```python
from build123d import *

# Parameters (mm, degrees)
SKETCH022_R        = 30
PAD_DEPTH          = 17
SKETCH023_R        = 0.7
POCKET_DEPTH       = 15.9
SKETCH024_R        = 0.55
POCKET001_DEPTH    = 13
SKETCH025_R        = 0.5
POCKET002_DEPTH    = 2
SKETCH026_W        = 5.1
SKETCH026_H        = 3.1
POCKET003_DEPTH    = 10
POLARPATTERN_COUNT = 3
SKETCH032_R        = 4
PAD002_DEPTH       = 7.5
SKETCH033_R        = 2.25
POCKET008_DEPTH    = 6
CHAMFER_SIZE       = 0.6
CHAMFER001_SIZE    = 0.8
SKETCH038_R        = 4.25
POCKET011_DEPTH    = 0.4
POCKET013_DEPTH    = 14
SKETCH046_W        = 4
SKETCH046_H        = 3
PAD010_DEPTH       = 14.5
CHAMFER006_SIZE    = 0.5
FILLET001_R        = 2


with BuildPart() as part:
    # Sketch022 (on DatumPlane) → Pad (new body)
    with BuildSketch(Plane(origin=(0, 0, -14.6), x_dir=(1, 0, 0), z_dir=(0, 0, -1))):
        Circle(SKETCH022_R)
    extrude(amount=PAD_DEPTH)

    # Sketch023 (on Face2 of Pad) → Pocket (cut)
    with BuildSketch(Plane.XY.offset(-14.6)):
        with Locations((-15, -15.2)):
            Circle(SKETCH023_R)
        with Locations((6.2, -16.6)):
            Circle(SKETCH023_R)
        with Locations((16.8, -8)):
            Circle(SKETCH023_R)
    extrude(amount=-POCKET_DEPTH, mode=Mode.SUBTRACT)

    # Sketch024 (on Face2 of Pocket) → Pocket001 (cut)
    with BuildSketch(Plane.XY.offset(-14.6)):
        with Locations((-11.85, -20.524803)):
            Circle(SKETCH024_R)
        with Locations((23.7, 0)):
            Circle(SKETCH024_R)
        with Locations((-11.85, 20.524802)):
            Circle(SKETCH024_R)
    extrude(amount=-POCKET001_DEPTH, mode=Mode.SUBTRACT)

    # Sketch025 (on Face2 of Pocket001) → Pocket002 (cut)
    with BuildSketch(Plane.XY.offset(-14.6)):
        with Locations((-16.1, 5.5)):
            Circle(SKETCH025_R)
        with Locations((-22.8, -6.4)):
            Circle(SKETCH025_R)
        with Locations((-15.5, -8.1)):
            Circle(SKETCH025_R)
        with Locations((-14.2, -12.7)):
            Circle(SKETCH025_R)
        with Locations((-14.6, -18.4)):
            Circle(SKETCH025_R)
        with Locations((-8.4, -22)):
            Circle(SKETCH025_R)
        with Locations((-5.2, -22.7)):
            Circle(SKETCH025_R)
        with Locations((3.6, -19.6)):
            Circle(SKETCH025_R)
        with Locations((6.2, -19.5)):
            Circle(SKETCH025_R)
        with Locations((10.240525, -14.05962)):
            Circle(SKETCH025_R)
        with Locations((23.6, 2.2)):
            Circle(SKETCH025_R)
        with Locations((16.4, 5.2)):
            Circle(SKETCH025_R)
    extrude(amount=-POCKET002_DEPTH, mode=Mode.SUBTRACT)

    # Sketch026 (on Face2 of Pocket002) → Pocket003 (cut)
    with BuildSketch(Plane.XY.offset(-14.6)):
        with Locations((0, -14.24549)):
            Rectangle(SKETCH026_W, SKETCH026_H)
    pocket003 = extrude(amount=-POCKET003_DEPTH, mode=Mode.SUBTRACT)

    # PolarPattern: Pocket003 ×3 about axis
    polarpattern_axis = Axis((0, 0, -14.6), (0, 0, 1))
    for i in range(1, POLARPATTERN_COUNT):
        add(pocket003.rotate(polarpattern_axis, i * 360 / POLARPATTERN_COUNT), mode=Mode.SUBTRACT)

    # Sketch032 (on Face2 of PolarPattern) → Pad002 (join)
    with BuildSketch(Plane.XY.offset(-14.6)):
        with Locations((12.5, 21.650635)):
            Circle(SKETCH032_R)
        with Locations((-25, 0)):
            Circle(SKETCH032_R)
        with Locations((12.5, -21.650635)):
            Circle(SKETCH032_R)
    extrude(amount=PAD002_DEPTH)

    # Sketch033 (on Face43 of Pad002) → Pocket008 (cut)
    with BuildSketch(Plane.XY.offset(-7.1)):
        with Locations((-25, 0)):
            Circle(SKETCH033_R)
        with Locations((12.5, 21.650635)):
            Circle(SKETCH033_R)
        with Locations((12.5, -21.650635)):
            Circle(SKETCH033_R)
    extrude(amount=-POCKET008_DEPTH, mode=Mode.SUBTRACT)

    # Chamfer
    chamfer_edges = [part.edges().sort_by_distance(p)[0] for p in [
        (-27.25, 0, -7.1),
        (10.25, -21.650635, -7.1),
        (10.25, 21.650635, -7.1),
    ]]
    chamfer(chamfer_edges, length=CHAMFER_SIZE)

    # Chamfer001
    chamfer001_edges = [part.edges().sort_by_distance(p)[0] for p in [
        (-29, 0, -14.6),
        (8.5, -21.650635, -14.6),
        (8.5, 21.650635, -14.6),
    ]]
    chamfer(chamfer001_edges, length=CHAMFER001_SIZE)

    # Sketch038 (on Face40 of Chamfer001) → Pocket011 (cut)
    with BuildSketch(Plane(origin=(0, 0, -31.6), x_dir=(1, 0, 0), z_dir=(0, 0, -1))):
        with Locations((-25, 0)):
            Circle(SKETCH038_R)
        with Locations((12.5, 21.650635)):
            Circle(SKETCH038_R)
        with Locations((12.5, -21.650635)):
            Circle(SKETCH038_R)
    extrude(amount=-POCKET011_DEPTH, mode=Mode.SUBTRACT)

    # Sketch045 (on Face4 of Pocket011) → Pocket013 (cut)
    with BuildSketch(Plane.XY.offset(-14.6)):
        with BuildLine():
            ThreePointArc((-7.25, 6.887489), (0, -10), (7.25, 6.887489))
            Line((7.25, 6.887489), (7.25, 30.887489))
            Line((7.25, 30.887489), (-7.25, 30.887489))
            Line((-7.25, 30.887489), (-7.25, 6.887489))
        make_face()
    extrude(amount=-POCKET013_DEPTH, mode=Mode.SUBTRACT)

    # Sketch046 (on Face9 of Pocket013) → Pad010 (join)
    with BuildSketch(Plane(origin=(7.25, 0, -14.6), x_dir=(0, 1, 0), z_dir=(-1, 0, 0))):
        with Locations((8.887489, 1.5)):
            Rectangle(SKETCH046_W, SKETCH046_H)
        with Locations((27.11078, 6.5)):
            Rectangle(SKETCH046_W, SKETCH046_H)
    extrude(amount=PAD010_DEPTH)

    # Chamfer006
    chamfer006_edges = [part.edges().sort_by_distance(p)[0] for p in [
        (23.15, 0, -14.6),
        (23.1, 2.2, -14.6),
        (15.9, 5.2, -14.6),
        (16.1, -8, -14.6),
        (9.740525, -14.05962, -14.6),
        (5.5, -16.6, -14.6),
        (5.7, -19.5, -14.6),
        (3.1, -19.6, -14.6),
        (-16.6, 5.5, -14.6),
        (-12.4, 20.524802, -14.6),
        (-16, -8.1, -14.6),
        (-14.7, -12.7, -14.6),
        (-15.7, -15.2, -14.6),
        (-15.1, -18.4, -14.6),
        (-12.4, -20.524803, -14.6),
        (-8.9, -22, -14.6),
        (-5.7, -22.7, -14.6),
        (-23.3, -6.4, -14.6),
    ]]
    chamfer(chamfer006_edges, length=CHAMFER006_SIZE)

    # Fillet001
    fillet001_edges = [part.edges().sort_by_distance(p)[0] for p in [
        (0, -10, -14.6),
        (0, 6.887489, -14.6),
    ]]
    fillet(fillet001_edges, radius=FILLET001_R)


solid = part.part
```
Check sheet for the modelled part. Datum: model origin and axes. Units: mm. A direction names the side the tool comes from. Round coordinates to 2 decimals unless told otherwise and drop trailing zeros. Loops run counter-clockwise (first coordinate to the right, second up) from the corner with the lowest first, then second, coordinate; pieces in that order, holes last. Notation, with made-up numbers: (-4, 60.25) -> (8, 60.25) arc R15 ccw to (8, 79.25) -> close; hole circle Ø8 at (-18.75, -33). An arc over 180 degrees is marked (long way). Answer in a Markdown table with one row per item.
Q1. Go/stop test with flat-tipped pins: P1, Ø10, axis at x = -6.5, y = -23.5, coming from the +Z side; P2, Ø0.5, axis at x = -16, y = 5.5, coming from the +Z side; P3, Ø1, axis at x = -8, z = -15, coming from the -Y side. Record where each tip stops, or that it passes through.
Data:
| item | result |
|---|---|
| P1 | stops at z = -14.6 |
| P2 | stops at z = -16.6 |
| P3 | stops at y = -29.05 |
Q2. Release check for a two-part mould opening along X. For faces 3 (the face through (-28.2, -2.4, -10.5)), 4 (the face through (0, 9, -17.6)) record: released by +X, released by -X, zero draft, split by the parting line, or undercut.
Data:
| item | result |
|---|---|
| face 3 | split by the parting line |
| face 4 | undercut |
Q3. Thickness scan on L1, parallel to Y at x = -25, z = -11; L2, parallel to Y at x = 12.5, z = -31.5; L3, parallel to Z at x = -8.5, y = -5. Record the ranges inside material, lowest first.
Data:
| item | result |
|---|---|
| L1 | y = -4 to -2.25, 2.25 to 4 |
| L2 | y = -27.27 to -25.9, -17.4 to 17.4, 25.9 to 27.27 |
| L3 | z = -31.6 to -28.6 |
Q4. Sectioned sample at B-B on y = 14. Enter the section's corners in (x, z), then the cut area to 3 significant figures.
Data:
| item | result |
|---|---|
| outline | (-26.53, -31.6) -> (26.53, -31.6) -> (26.53, -14.6) -> (7.25, -14.6) -> (7.25, -28.6) -> (-7.25, -28.6) -> (-7.25, -14.6) -> (-26.53, -14.6) -> close |
| area | 699 mm^2 |
Q5. Sectioned sample at A-A on z = -10. Enter the section's corners in (x, y), then the cut area to 3 significant figures.
Data:
| item | result |
|---|---|
| outline | circle Ø8 at (-25, 0); circle Ø8 at (12.5, -21.65); circle Ø8 at (12.5, 21.65); hole circle Ø4.5 at (-25, 0); hole circle Ø4.5 at (12.5, -21.65); hole circle Ø4.5 at (12.5, 21.65) |
| area | 103 mm^2 |
Q6. Set-up check for faces 1 (the face through (12, 7, -24.6)), 2 (the face through (11.58, 25.8, -31.4)): record each of +Z, -Z, +X, -X, +Y, -Y from which the full face is reachable in a straight line by a thin tool's end or side.
Data:
| item | result |
|---|---|
| face 1 | +Z |
| face 2 | -Z |
